Input: dimensioned drawing with shaded views. Units: mm. Origin: part minimum x, y, z. A direction names the side the tool comes from. Give positions to 0.01 mm unless a question says otherwise; leave off trailing zeros. Order: outer loops, then holes, each group sorted by start corner. A loop starts at its lowest first (then second) coordinate and runs counter-clockwise, first axis right, second up.
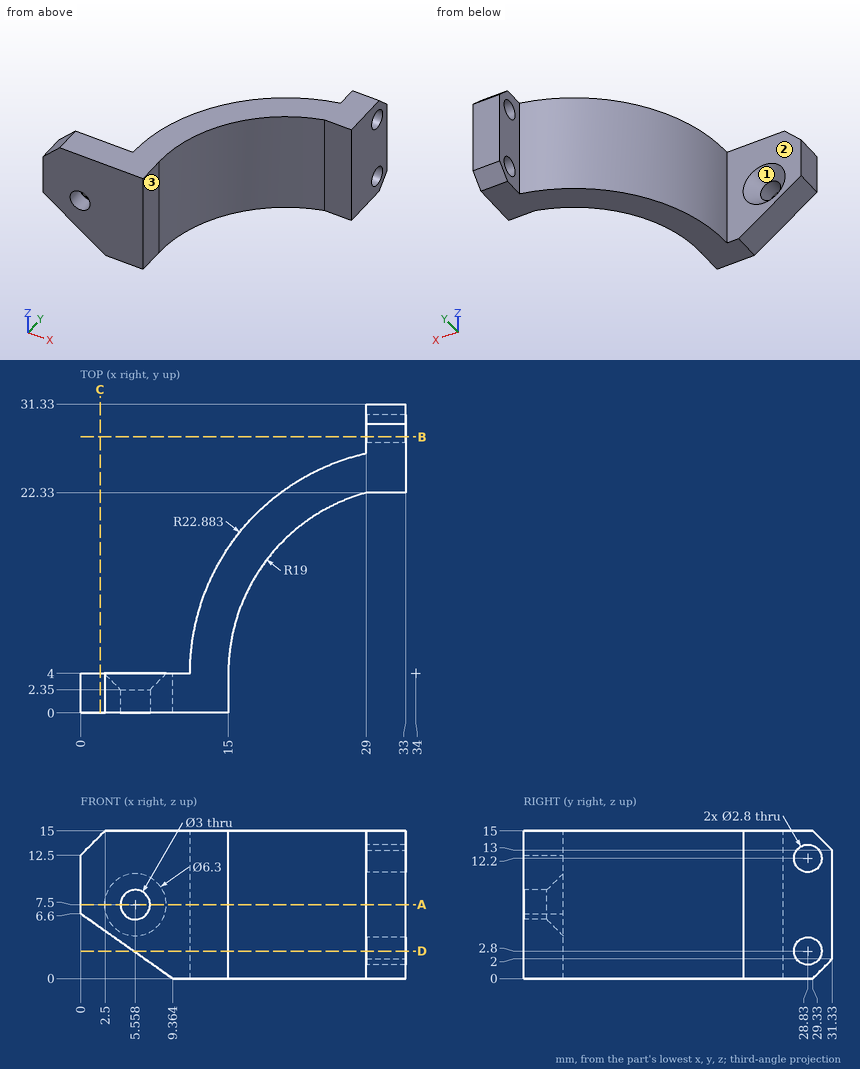
1) Section query A-A, the plane z = 7.5. Return the cut outline in (x, y).
Report:
outline: (0, 0) - (4.06, 0) - (4.06, 2.35) - (2.41, 4) - (0, 4) - close; (7.06, 0) - (15, 0) - (15, 4) arc R19 cw to (29, 22.33) - (33, 22.33) - (33, 31.33) - (29, 31.33) - (29, 26.33) arc R22.88 ccw to (11.12, 4) - (8.71, 4) - (7.06, 2.35) - close
2) Section query C-C, the plane x = 2. Return the cut outline in (y, z).
Report:
outline: (0, 5.19) - (4, 5.19) - (4, 14.5) - (0, 14.5) - close
3) Section query B-B, the plane y = 28. Return the cut outline in (x, z).
Report:
outline: (29, 0) - (33, 0) - (33, 1.67) - (29, 1.67) - close; (29, 3.93) - (33, 3.93) - (33, 11.07) - (29, 11.07) - close; (29, 13.33) - (33, 13.33) - (33, 15) - (29, 15) - close
4) Material intervals for L1, parallel to Y at x = 6, z = 9 (1 decimal); L2, parallel to Y at x = 23.5, z = 10 (1 decimal); L3, parallel to X at y = 18, z = 7.5 (1 decimal), sorted ascending.
Report:
L1: y = 0 to 2.4
L2: y = 19.8 to 24.3
L3: x = 15.9 to 21.2
5) Section query D-D, the plane z = 2.8. Return the cut outline in (x, y).
Report:
outline: (5.39, 0) - (15, 0) - (15, 4) arc R19 cw to (29, 22.33) - (33, 22.33) - (33, 27.43) - (29, 27.43) - (29, 26.33) arc R22.88 ccw to (11.12, 4) - (5.39, 4) - close; (29, 30.23) - (33, 30.23) - (33, 31.33) - (29, 31.33) - close
6) Reachability of the marked faces 1, 2 and 3 from +Z, -Z, +X, -X, +Y, -Y: full face, straight path, thin tool, end or side. Return the list, or none.
Report:
face 1: +Y
face 2: +Z, -Z, -X, +Y
face 3: +Z, -Z, +X, -Y
7) Pin query (flat end, axial travel): pin 1 (3 mm diameter, centred on x = 8.5, y = 10.5, fed in from -Z); pin 2 (1.2 mm diameter, centred on x = 30.5, z = 4, fed in from -Y); pin 3 (5.5 mm diameter, centred on x = 4.5, z = 10.5, fed in from +Y); pin 4 (1.5 mm diameter, centred on y = 29, z = 5.5, fed in from -X). Return the tip coordinate at first contact, or that it passes through.
Report:
pin 1: passes through
pin 2: stops at y = 22.33
pin 3: stops at y = 4
pin 4: stops at x = 29
